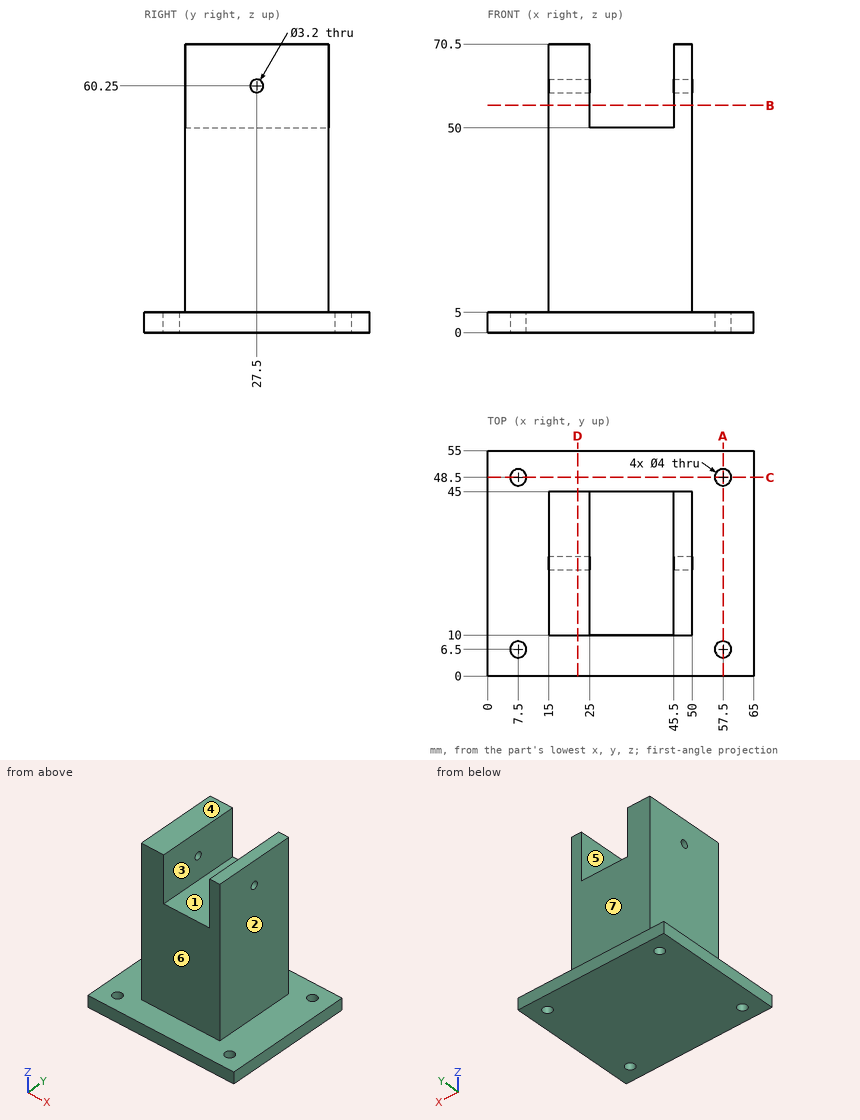
Source: three-view drawing plus pictorial views. Frame: mm from the lowest corner of the part. A direction names the side the tool comes from. Round coordinates to 2 decimals unless told otherwise and drop trailing zeros. Loops run counter-clockwise (first coordinate to the right, second up) from the corner with the lowest first, then second, coordinate; pieces in that order, holes last.
Q1. Mould query, pull axis X, two halves, no side actions, for the marked faces 1, 2, 3 and 4. Classes: pulls with the +X half, pulls with the -X half, needs draft (parallel to the pull), parting line crosses it, or undercut.
Q2. Section A-A, the plane x = 57.5. Return loops of the section in (y, z).
Q3. First-contact query: P1, Ø3.5, axis at x = 7.5, y = 48.5, coming from the +Z side; P2, Ø4, axis at y = 33, z = 34.5, coming from the +X side; P3, Ø17.5, axis at x = 32.5, z = 25.5, coming from the -Y side; P4, Ø4, axis at y = 9.5, z = 21, coming from the -X side. Flat tips, straight axial feed; report the tip coordinate or a pass-through.
Q4. Access query for the marked faces 5, 6 and 7. Directions: +Z, -Z, +X, -X, +Y, -Y. A direction counts if a zero-diameter tool reaches every point of the face in a straight line with its end or side. Return the directions, or none.
Q5. Section D-D, the plane x = 22. Return loops of the section in (y, z), plus the area to 3 significant figures.
Q6. Section C-C, the plane y = 48.5. Return loops of the section in (x, z).
Q7. Ray query, line 1 (Y direction, x = 7.5, z = 1.4); line 2 (X direction, y = 6, z = 1); line 3 (X direction, y = 24, z = 59.5). Return the intervals inside material, ascending.
Q8. Section B-B, the plane z = 55.5. Return loops of the section in (x, y).
Solutions:
1. face 1: undercut
1. face 2: pulls with the +X half
1. face 3: undercut
1. face 4: needs draft
2. outline: (0, 0) - (4.5, 0) - (4.5, 5) - (0, 5) - close; (8.5, 0) - (46.5, 0) - (46.5, 5) - (8.5, 5) - close; (50.5, 0) - (55, 0) - (55, 5) - (50.5, 5) - close
3. P1: passes through
3. P2: stops at x = 50
3. P3: stops at y = 10
3. P4: stops at x = 15
4. face 5: +Z, +Y, -Y
4. face 6: +Z, +X, -X, -Y
4. face 7: +Z, +X, -X, +Y
5. outline: (0, 0) - (55, 0) - (55, 5) - (45, 5) - (45, 70.5) - (10, 70.5) - (10, 5) - (0, 5) - close; hole circle Ø3.2 at (27.5, 60.25)
5. area: 2,560 mm2
6. outline: (0, 0) - (5.5, 0) - (5.5, 5) - (0, 5) - close; (9.5, 0) - (55.5, 0) - (55.5, 5) - (9.5, 5) - close; (59.5, 0) - (65, 0) - (65, 5) - (59.5, 5) - close
7. line 1: y = 0 to 4.5, 8.5 to 46.5, 50.5 to 55
7. line 2: x = 0 to 5.56, 9.44 to 55.56, 59.44 to 65
7. line 3: x = 15 to 25, 45.5 to 50
8. outline: (15, 10) - (25, 10) - (25, 45) - (15, 45) - close; (45.5, 10) - (50, 10) - (50, 45) - (45.5, 45) - close
